```python
from build123d import *

# Parameters (mm, degrees)
BOSS_EXTRUDE1_DEPTH = 60
SKETCH2_R           = 25
CUT_EXTRUDE1_DEPTH  = 5.5
FILLET1_SIZE        = 12
FILLET1_SIZE_2      = 20
FILLET2_SIZE        = 20
FILLET2_SIZE_2      = 12
FILLET3_SIZE        = 20
FILLET3_SIZE_2      = 12
SKETCH4_R           = 20.5
CUT_EXTRUDE2_DEPTH  = 8.5
SKETCH6_R           = 28
CUT_EXTRUDE3_DEPTH  = 5.973425633


with BuildPart() as part:
    # Sketch1 → Boss-Extrude1 (new body)
    with BuildSketch(Plane(origin=(0, 0, 0), x_dir=(1, 0, 0), z_dir=(0, 1, 0))):
        Polygon((-44.639505024, 1.864709672), (-31.939505024, 1.864709672), (-31.939505024, -4.108715961), (31.939505024, -4.108715961), (31.939505024, 1.864709672), (44.639505024, 1.864709672), (44.639505024, 5.364709672), (-44.639505024, 5.364709672), align=None)
    extrude(amount=BOSS_EXTRUDE1_DEPTH)

    # Sketch2 → Cut-Extrude1 (cut)
    with BuildSketch(Plane(origin=(0, 0, -5.364709672), x_dir=(-1, 0, 0), z_dir=(0, 0, -1))):
        with Locations((0, 30)):
            Circle(SKETCH2_R)
    extrude(amount=-CUT_EXTRUDE1_DEPTH, mode=Mode.SUBTRACT)

    # Fillet1
    # an asymmetric fillet: 20, 12 mm, written as the material it takes off along each edge
    with BuildSketch(Plane(origin=(-44.639505024, 60, -55.364709672), x_dir=(0, -1, 0), z_dir=(0, 0, 1))) as fillet1_piece_1:
        with BuildLine():
            Bezier((FILLET1_SIZE, 0), (0, 0), (0, FILLET1_SIZE_2), weights=[1, 0.707106781, 1])
            Line((0, FILLET1_SIZE_2), (0, 0))
            Line((0, 0), (FILLET1_SIZE, 0))
        make_face()
    extrude(amount=103.5, mode=Mode.SUBTRACT)
    with BuildSketch(Plane(origin=(44.639505024, 60, 48.135290328), x_dir=(-1, 0, 0), z_dir=(0, 0, -1))) as fillet1_piece_2:
        with BuildLine():
            Bezier((FILLET1_SIZE_2, 0), (0, 0), (0, -FILLET1_SIZE), weights=[1, 0.707106781, 1])
            Line((0, -FILLET1_SIZE), (0, 0))
            Line((0, 0), (FILLET1_SIZE_2, 0))
        make_face()
    extrude(amount=103.5, mode=Mode.SUBTRACT)

    # Fillet2
    # an asymmetric fillet: 20, 12 mm, written as the material it takes off along each edge
    with BuildSketch(Plane(origin=(44.639505024, 0, 48.135290328), x_dir=(-1, 0, 0), z_dir=(0, 0, -1))) as fillet2_piece_1:
        with BuildLine():
            Bezier((FILLET2_SIZE, 0), (0, 0), (0, FILLET2_SIZE_2), weights=[1, 0.707106781, 1])
            Line((0, FILLET2_SIZE_2), (0, 0))
            Line((0, 0), (FILLET2_SIZE, 0))
        make_face()
    extrude(amount=103.5, mode=Mode.SUBTRACT)

    # Fillet3
    # an asymmetric fillet: 20, 12 mm, written as the material it takes off along each edge
    with BuildSketch(Plane(origin=(-44.639505024, 0, -55.364709672), x_dir=(1, 0, 0), z_dir=(0, 0, 1))) as fillet3_piece_1:
        with BuildLine():
            Bezier((FILLET3_SIZE, 0), (0, 0), (0, FILLET3_SIZE_2), weights=[1, 0.707106781, 1])
            Line((0, FILLET3_SIZE_2), (0, 0))
            Line((0, 0), (FILLET3_SIZE, 0))
        make_face()
    extrude(amount=103.5, mode=Mode.SUBTRACT)

    # Sketch4 → Cut-Extrude2 (cut)
    with BuildSketch(Plane(origin=(0, 0, 0.135290328), x_dir=(-1, 0, 0), z_dir=(0, 0, -1))):
        with Locations((0, 30)):
            Circle(SKETCH4_R)
    extrude(amount=-CUT_EXTRUDE2_DEPTH, mode=Mode.SUBTRACT)

    # Sketch6 → Cut-Extrude3 (cut)
    with BuildSketch(Plane.XY.offset(4.108715961)):
        with BuildLine():
            Line((-31.939505024, 59.172090225), (-31.939505024, 0.827909775))
            add(Edge.make_bspline(
                [(-31.939505024, 0.827909775), (-28.419914948, -2e-09), (-24.63950501, 0)],
                knots=[0, 0, 0, 1, 1, 1], degree=2))
            Line((-24.63950501, 0), (24.639505024, 0))
            add(Edge.make_bspline(
                [(24.639505024, 0), (28.419914955, 0), (31.939505024, 0.827909775)],
                knots=[0, 0, 0, 1, 1, 1], degree=2))
            Line((31.939505024, 0.827909775), (31.939505024, 59.172090225))
            add(Edge.make_bspline(
                [(31.939505024, 59.172090225), (28.419914948, 60.000000002), (24.63950501, 60)],
                knots=[0, 0, 0, 1, 1, 1], degree=2))
            Line((24.63950501, 60), (-24.639505024, 60))
            add(Edge.make_bspline(
                [(-24.639505024, 60), (-28.419914955, 60), (-31.939505024, 59.172090225)],
                knots=[0, 0, 0, 1, 1, 1], degree=2))
        make_face()
        with Locations((0, 30)):
            Circle(SKETCH6_R, mode=Mode.SUBTRACT)
    extrude(amount=-CUT_EXTRUDE3_DEPTH, mode=Mode.SUBTRACT)


solid = part.part
```
Design review of the part built by this model. Coordinates are the model's own, in mm. A direction names the side the tool comes from. Coordinates: 2 decimals unless noted, no trailing zeros. Write each loop counter-clockwise with the first axis right and the second up, starting at its lowest first coordinate (ties: lowest second). Pieces come first, ordered by that corner, then holes. Notation, with made-up numbers: M 73,44.5 L 83,44.5 A20 cw 83,61.5 Z; hole C -32,83 d10. An arc over 180 degrees is marked long. Answer as a JSON object with one key per item and string values.
Item 1: Wall thickness on probe 1 along Y at (x, z) = (0, 2.85); probe 2 along Y at (x, z) = (-0.5, -1.5) (3 decimals); probe 3 along Z at (x, y) = (9, 7): over which ranges is each line inside the solid? List them lowest first.
Outcome:
{"probe 1": "2 to 9.5, 50.5 to 58", "probe 2": "2.004 to 5.005, 54.995 to 57.996", "probe 3": "0.14 to 4.11"}
Item 2: Machinability: for faces 1 (the flat face through (0, 0, -4)), 2 (the cylindrical face through (-6.07, 2.666, 1.164)), which of the approach directions +Z, -Z, +X, -X, +Y, -Y give a long, thin tool a straight path to every point of the face, cutting with its end or side? Answer none if there is none.
Outcome:
{"face 1": "+Z, -Z, +X, -X, -Y", "face 2": "+Z"}
Item 3: Insertion check: pin 1 Ø3 at (y, z) = (22.5, 0) entering from +X; pin 2 Ø1 at (x, y) = (34, 30.5) entering from +Z; pin 3 Ø1.5 at (y, z) = (8, -2) entering from +X. Each pin has a flat end and moves straight along its axis. Give the tip position at first contact, or say it passes through.
Outcome:
{"pin 1": "x = 27.35", "pin 2": "z = -1.86", "pin 3": "x = 43.89"}
Item 4: Draft analysis for pull direction X (two halves, no side actions). For faces 3 (the cylindrical face through (-11.5, 7.8, -2.7)), 4 (the flat face through (3.8, 50.5, 0.135)), 5 (the flat face through (44.64, 30, -4)), 6 (the flat face through (1, 56, -5.365)), state which applies: pulls with the +X half, pulls with the -X half, needs draft (parallel to the pull), parting line crosses it, or undercut.
Outcome:
{"face 3": "undercut", "face 4": "undercut", "face 5": "pulls with the +X half", "face 6": "needs draft"}
Item 5: Add section D-D, the plane x = -22.5. Give the boundary of the cut face in (y, z), and give its area (3 significant figures).
Outcome:
{"outline": "M 0,-5.36 L 19.1,-5.36 L 19.1,0.14 L 40.9,0.14 L 40.9,-5.36 L 60,-5.36 L 60,-1.86 L 46.67,-1.86 L 46.67,4.11 L 13.33,4.11 L 13.33,-1.86 L 0,-1.86 Z", "area": "289 mm²"}
Item 6: Add section B-B, the plane x = 0. Give the boundary of the cut face in (y, z).
Outcome:
{"outline": "M 0,-5.36 L 5,-5.36 L 5,0.14 L 9.5,0.14 L 9.5,4.11 L 2,4.11 L 2,-1.86 L 0,-1.86 Z; M 50.5,0.14 L 55,0.14 L 55,-5.36 L 60,-5.36 L 60,-1.86 L 58,-1.86 L 58,4.11 L 50.5,4.11 Z"}
Item 7: Add section A-A, the plane y = 30. Give the boundary of the cut face in (x, z), and give its area (3 significant figures).
Outcome:
{"outline": "M -44.64,-5.36 L -25,-5.36 L -25,0.14 L -20.5,0.14 L -20.5,4.11 L -28,4.11 L -28,-1.86 L -44.64,-1.86 Z; M 20.5,0.14 L 25,0.14 L 25,-5.36 L 44.64,-5.36 L 44.64,-1.86 L 28,-1.86 L 28,4.11 L 20.5,4.11 Z", "area": "209 mm²"}
Item 8: Add section C-C, the plane z = 1.25. Give the boundary of the cut face in (x, y).
Outcome:
{"outline": "C 0,30 d56; hole C 0,30 d41"}
